Check sheet for the modelled part. Datum: model origin and axes. Units: mm. A direction names the side the tool comes from. Coordinates: 2 decimals unless noted, no trailing zeros. Write each loop counter-clockwise with the first axis right and the second up, starting at its lowest first coordinate (ties: lowest second). Pieces come first, ordered by that corner, then holes. Notation, with made-up numbers: (3, -21.5) - (39, -21.5) arc R23 cw to (39, 8.5) - close; hole circle Ø2 at (-15, 46.25). An arc over 180 degrees is marked (long way). Write each question's results on one line, items separated by ' | '.
from build123d import *

# Parameters (mm, degrees)
F1_DEPTH = 63.5
F2_DEPTH = 25.4
F3_DEPTH = 7.9375
F5_R     = 6.35


with BuildPart() as f1:
    # F0 (on Front) → F1 (new body, symmetric)
    with BuildSketch(Plane.XZ):
        Polygon((-41.275, -9.525), (41.275, -9.525), (41.275, 9.525), (22.225, 9.525), (-41.275, 9.525), align=None)
    extrude(amount=F1_DEPTH, both=True)

    # F0 (on Front) → F2 (join, symmetric)
    with BuildSketch(Plane.XZ):
        Polygon((86.0701791132, 61.9252), (60.325, 61.9252), (60.325, 42.8752), (85.7941830205, 42.8752), align=None)
        with BuildLine():
            Line((22.225, 9.525), (41.275, 9.525))
            Line((41.275, 9.525), (41.275, 27.0002))
            ThreePointArc((41.275, 27.0002), (45.9246798487, 38.2255201513), (57.15, 42.8752))
            Line((57.15, 42.8752), (60.325, 42.8752))
            Line((60.325, 42.8752), (60.325, 61.9252))
            Line((60.325, 61.9252), (57.15, 61.9252))
            ThreePointArc((57.15, 61.9252), (32.4542956671, 51.6959043329), (22.225, 27.0002))
            Line((22.225, 27.0002), (22.225, 9.525))
        make_face()
    extrude(amount=F2_DEPTH, both=True)

    # F0 (on Front) → F3 (join, symmetric)
    with BuildSketch(Plane.XZ):
        with BuildLine():
            add(Edge.make_bspline(
                [(-41.275, 9.525), (-31.1370120476, 45.302397555), (-2.1070703483, 62.4784893272), (57.15, 61.9252)],
                knots=[0, 0, 0, 0, 111.5045361635, 111.5045361635, 111.5045361635, 111.5045361635], degree=3))
            Line((-41.275, 9.525), (22.225, 9.525))
            Line((22.225, 9.525), (22.225, 27.0002))
            ThreePointArc((22.225, 27.0002), (32.4542956671, 51.6959043329), (57.15, 61.9252))
        make_face()
    extrude(amount=F3_DEPTH, both=True)

    # F0 (on Front) → F4 (revolve)
    with BuildSketch(Plane.XZ):
        Polygon((86.1389941389, 66.675), (86.0701791132, 61.9252), (85.7941830205, 42.8752), (85.725, 38.1), (111.125, 38.1), (111.125, 66.675), align=None)
    revolve(axis=Axis((85.9319970695, 0, 52.3875), (0.0144864636, 0, 0.9998950657)))

    # F5
    f5_edges = [f1.edges().sort_by_distance(p)[0] for p in [
        (41.275, -63.5, 0),
        (-41.275, -63.5, 0),
        (-41.275, 63.5, 0),
        (41.275, 63.5, 0),
    ]]
    fillet(f5_edges, radius=F5_R)


solid = f1.part
1. Material ranges on L1, parallel to X at y = 22.5, z = 14.5 (3 decimals); L2, parallel to Z at x = 70.5, y = 24; L3, parallel to Y at x = -1, z = 19, recorded low to high. Write a range as [from, to].
Values follow:
L1: x = [22.225, 41.275] | L2: z = [42.88, 61.93] | L3: y = [-7.94, 7.94]
2. Draft check along X on faces 1 (the flat face through (60, 0, 42.875)), 2 (the flat face through (0, -63.5, 0)), 3 (the cylindrical face through (-39.464, -61.59, -0.133)). Enter one of: pulls with the +X half, pulls with the -X half, needs draft (parallel to the pull), parting line crosses it, or undercut.
Values follow:
face 1: undercut | face 2: needs draft | face 3: pulls with the -X half
3. Access from +Z, -Z, +X, -X, +Y, -Y to the whole of each face (thin tool, end or side, straight path). Record for faces 4 (the flat face through (47, -25.4, 42)), 5 (the flat face through (-2, 7.938, 30)), 6 (the conical face through (87.296, 0.364, 66.676)).
Values follow:
face 4: +Z, +X, -X, -Y | face 5: +Z, -X, +Y | face 6: +Z, +X
4. Sectioned sample at A-A (y = -41). Record the cut outline in (x, z) (3 decimals).
Values follow:
outline: (-41.275, -9.525) - (41.275, -9.525) - (41.275, 9.525) - (-41.275, 9.525) - close
5. Go/stop test with flat-tipped pins: pin 1 (14 mm diameter, centred on y = 13, z = 22.5, fed in from -X); pin 2 (6 mm diameter, centred on x = 36, y = 4, fed in from +Z); pin 3 (5 mm diameter, centred on x = 84.5, y = 23.5, fed in from -Z). Record where each tip stops, or that it passes through.
Values follow:
pin 1: stops at x = -38.51 | pin 2: stops at z = 61.48 | pin 3: stops at z = 38.41
